Build history of the part. All positions in model axes, mm. Face numbers are marked on the shaded views. A direction names the side the tool comes from. Round coordinates to 2 decimals unless told otherwise and drop trailing zeros. Loops run counter-clockwise (first coordinate to the right, second up) from the corner with the lowest first, then second, coordinate; pieces in that order, holes last. Notation, with made-up numbers: (3.5, 85.25) - (44.5, 85.25) arc R32 cw to (44.5, 117.25) - close; hole circle Ø7 at (18, 64.25). An arc over 180 degrees is marked (long way). Put each result on its own line as item: value. Start each with the question number.
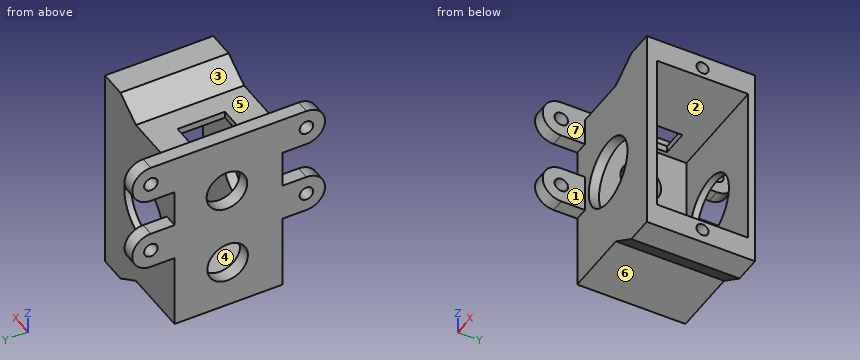
from build123d import *

# Parameters (mm, degrees)
P_IDAT_VYSUNUT_M1_DEPTH   = 15
P_IDAT_VYSUNUT_M2_DEPTH   = 15
SKICA10_W                 = 16
SKICA10_H                 = 24
ODEBRAT_VYSUNUT_M7_DEPTH  = 13.5
SKICA11_W                 = 2.5
SKICA11_H                 = 15
P_IDAT_VYSUNUT_M3_DEPTH   = 4
SKICA12_R                 = 0.9
ODEBRAT_VYSUNUT_M8_DEPTH  = 4
SKICA13_W                 = 4
SKICA13_H                 = 7
ODEBRAT_VYSUNUT_M9_DEPTH  = 4
SKICA17_W                 = 38.25
SKICA17_H                 = 32.5
ODEBRAT_VYSUNUT_M10_DEPTH = 16
P_IDAT_VYSUNUT_M4_DEPTH   = 1
SKICA20_R                 = 1
P_IDAT_VYSUNUT_M5_DEPTH   = 2
SKICA21_R                 = 5
ODEBRAT_VYSUNUT_M11_DEPTH = 22
LINPOLE1_COUNT            = 2
LINPOLE1_PITCH            = 11
SKICA22_R                 = 3
ODEBRAT_VYSUNUT_M12_DEPTH = 5
P_IDAT_VYSUNUT_M6_DEPTH   = 16
SKICA24_W                 = 2
SKICA24_H                 = 1.5
P_IDAT_VYSUNUT_M7_DEPTH   = 16


with BuildPart() as part:
    # Skica1 → Přidat vysunutím1 (new body)
    with BuildSketch(Plane(origin=(0, 0, 0), x_dir=(1, 0, 0), z_dir=(0, 1, 0))):
        Polygon((0, -11), (0, 11), (-3.25, 14.25), (-30.25, 14.25), (-30.25, 16.25), (-2.421572875, 16.25), (2, 11.828427125), (2, -11.828427125), (-2.421572875, -16.25), (-30.25, -16.25), (-30.25, -14.25), (-3.25, -14.25), align=None)
    extrude(amount=P_IDAT_VYSUNUT_M1_DEPTH)

    # Skica8 → Přidat vysunutím2 (add)
    with BuildSketch(Plane.XZ):
        Polygon((-0.343145751, 14.171572875), (26, 14.171572875), (26, -11.828427125), (2, -11.828427125), (2, 11.828427125), align=None)
    extrude(amount=-P_IDAT_VYSUNUT_M2_DEPTH)

    # Skica10 → Odebrat vysunutím7 (cut)
    with BuildSketch(Plane(origin=(0, 15, 0), x_dir=(1, 0, 0), z_dir=(0, 1, 0))):
        with Locations((18, -1.171572875)):
            Rectangle(SKICA10_W, SKICA10_H)
    extrude(amount=-ODEBRAT_VYSUNUT_M7_DEPTH, mode=Mode.SUBTRACT)

    # Skica11 → Přidat vysunutím3 (add)
    with BuildSketch(Plane(origin=(26, 0, 0), x_dir=(0, 0, -1), z_dir=(1, 0, 0))):
        with Locations((-15.421572875, 7.5)):
            Rectangle(SKICA11_W, SKICA11_H)
        with Locations((13.078427125, 7.5)):
            Rectangle(SKICA11_W, SKICA11_H)
    extrude(amount=-P_IDAT_VYSUNUT_M3_DEPTH)

    # Skica12 → Odebrat vysunutím8 (cut)
    with BuildSketch(Plane(origin=(26, 0, 0), x_dir=(0, 0, -1), z_dir=(1, 0, 0))):
        with Locations((-14.730217843, 8.25)):
            Circle(SKICA12_R)
        with Locations((12.269782157, 8.25)):
            Circle(SKICA12_R)
    extrude(amount=-ODEBRAT_VYSUNUT_M8_DEPTH, mode=Mode.SUBTRACT)

    # Skica13 → Odebrat vysunutím9 (cut)
    with BuildSketch(Plane.XY.offset(14.171572875)):
        with Locations((12.656854249, 8.25)):
            Rectangle(SKICA13_W, SKICA13_H)
    extrude(amount=-ODEBRAT_VYSUNUT_M9_DEPTH, mode=Mode.SUBTRACT)

    # Skica17 → Odebrat vysunutím10 (cut, through all)
    with BuildSketch(Plane(origin=(0, 15, 0), x_dir=(1, 0, 0), z_dir=(0, 1, 0))):
        with Locations((-11.125, 0)):
            Rectangle(SKICA17_W, SKICA17_H)
    extrude(amount=-ODEBRAT_VYSUNUT_M10_DEPTH, mode=Mode.SUBTRACT)

    # Skica19 → Přidat vysunutím4 (add)
    with BuildSketch(Plane(origin=(0, 15, 0), x_dir=(1, 0, 0), z_dir=(0, 1, 0))):
        Polygon((8, 11.828427125), (22, 11.828427125), (22, 14.328427125), (26, 14.328427125), (26, -16.671572875), (22, -16.671572875), (22, -14.171572875), (8, -14.171572875), align=None)
    extrude(amount=P_IDAT_VYSUNUT_M4_DEPTH)

    # Skica20 → Přidat vysunutím5 (add)
    with BuildSketch(Plane.ZY.offset(-8)):
        with BuildLine():
            Line((10.171572875, -3.5), (10.171572875, 0))
            Line((10.171572875, 0), (15.671572875, 0))
            Line((15.671572875, 0), (15.671572875, -3.5))
            ThreePointArc((15.671572875, -3.5), (12.921572875, -6.25), (10.171572875, -3.5))
        make_face()
        with Locations((12.921572875, -3.5)):
            Circle(SKICA20_R, mode=Mode.SUBTRACT)
        with BuildLine():
            Line((10.171572875, 16), (15.671572875, 16))
            Line((15.671572875, 16), (15.671572875, 19.5))
            ThreePointArc((15.671572875, 19.5), (12.921572875, 22.25), (10.171572875, 19.5))
            Line((10.171572875, 19.5), (10.171572875, 16))
        make_face()
        with Locations((12.921572875, 19.5)):
            Circle(SKICA20_R, mode=Mode.SUBTRACT)
    p_idat_vysunut_m5 = extrude(amount=-P_IDAT_VYSUNUT_M5_DEPTH)

    # Skica21 → Odebrat vysunutím11 (cut)
    with BuildSketch(Plane(origin=(0, 16, 0), x_dir=(1, 0, 0), z_dir=(0, 1, 0))):
        with Locations((16, -1.171572875)):
            Circle(SKICA21_R)
    extrude(amount=-ODEBRAT_VYSUNUT_M11_DEPTH, mode=Mode.SUBTRACT)

    # LinPole1: Přidat vysunutím5 ×2
    with Locations(*[(0, 0, -i * LINPOLE1_PITCH) for i in range(1, LINPOLE1_COUNT)]):
        add(p_idat_vysunut_m5)

    # Skica22 → Odebrat vysunutím12 (cut)
    with BuildSketch(Plane(origin=(10, 0, 0), x_dir=(0, 0, -1), z_dir=(1, 0, 0))):
        with Locations((-7.230444291, 8.25)):
            Circle(SKICA22_R)
        with Locations((4.769102832, 8.145746213)):
            Circle(SKICA22_R)
    extrude(amount=-ODEBRAT_VYSUNUT_M12_DEPTH, mode=Mode.SUBTRACT)

    # Skica23 → Přidat vysunutím6 (add)
    with BuildSketch(Plane(origin=(0, 16, 0), x_dir=(1, 0, 0), z_dir=(0, 1, 0))):
        Polygon((22, 14.328427125), (18, 11.828427125), (22, 11.828427125), align=None)
        Polygon((22, -14.171572875), (18, -14.171572875), (22, -16.671572875), align=None)
    extrude(amount=-P_IDAT_VYSUNUT_M6_DEPTH)

    # Skica24 → Přidat vysunutím7 (add)
    with BuildSketch(Plane.XZ.offset(-16)):
        with Locations((9, 14.921572875)):
            Rectangle(SKICA24_W, SKICA24_H)
    extrude(amount=P_IDAT_VYSUNUT_M7_DEPTH)


solid = part.part
Item 1: Which spindle directions (+Z, -Z, +X, -X, +Y, -Y) get a long thin tool onto all of the face, cutting with end or side? Do the marked faces 4, 5, 6 and 7. Say none if no direction does.
Item 2: Slice it at B-B (x = 16). Give the cut face in (y, z).
Item 3: Two-plate mould, pull along X, no slides. Class the marked faces 1, 2 and 3: pulls with the +X half, pulls with the -X half, needs draft (parallel to the pull), parting line crosses it, or undercut.
Item 4: Slice it at D-D (x = 13.5). Give the cut face in (y, z), plus the area to 3 significant figures.
Item 5: Slice it at A-A (x = 23). Give the cut face in (y, z).
Item 6: Drop flat-ended pins along their axis: pin 1 Ø2 at (x, y) = (9, -1.5) entering from +Z; pin 2 Ø10 at (x, z) = (20, 6.5) entering from +Y; pin 3 Ø2 at (y, z) = (8, -12.5) entering from +X; pin 4 Ø8 at (x, y) = (12, 8.5) entering from -Z. Give the stop position or say it passes through.
Item 7: Slice it at C-C (z = 11). Give the cut face in (x, y), plus the area to 3 significant figures.
Item 8: Drill centre lines: probe 1 along Z at (x, y) = (23.95, 8.25); probe 2 along Z at (x, y) = (25, 9.25); probe 3 along Z at (x, y) = (12.75, 13). Where is each one in solid material? Low to high. Write a range as [from, to].
Computed values:
1. face 4: +X
1. face 5: +Z, +Y, -Y
1. face 6: -Z, -X, +Y, -Y
1. face 7: +Z
2. outline: (0, -11.83) - (16, -11.83) - (16, -3.83) - (15, -3.83) - (15, -10.83) - (1.5, -10.83) - (1.5, -3.83) - (0, -3.83) - close; (0, 6.17) - (1.5, 6.17) - (1.5, 13.17) - (15, 13.17) - (15, 6.17) - (16, 6.17) - (16, 14.17) - (0, 14.17) - close
3. face 1: pulls with the +X half
3. face 2: needs draft
3. face 3: undercut
4. outline: (0, -11.83) - (16, -11.83) - (16, -3.16) - (15, -3.16) - (15, -10.83) - (1.5, -10.83) - (1.5, -3.16) - (0, -3.16) - close; (0, 5.5) - (1.5, 5.5) - (1.5, 13.17) - (4.75, 13.17) - (4.75, 14.17) - (0, 14.17) - close; (11.75, 13.17) - (15, 13.17) - (15, 5.5) - (16, 5.5) - (16, 14.17) - (11.75, 14.17) - close
4. area: 63.3 mm^2
5. outline: (0, -14.33) - (16, -14.33) - (16, 16.67) - (0, 16.67) - close; hole (1.5, -10.83) - (15, -10.83) - (15, 13.17) - (1.5, 13.17) - close; hole circle Ø1.8 at (8.25, -12.27); hole circle Ø1.8 at (8.25, 14.73)
6. pin 1: stops at z = 15.67
6. pin 2: stops at y = 16
6. pin 3: stops at x = 26
6. pin 4: stops at z = -11.83
7. outline: (8, -5.47) - (10, -5.47) - (10, 0) - (26, 0) - (26, 1.5) - (10, 1.5) - (10, 15) - (26, 15) - (26, 16) - (10, 16) - (10, 21.47) - (8, 21.47) - close
7. area: 93.9 mm^2
8. probe 1: z = [-14.33, -13.17], [-11.37, -10.83], [13.17, 13.83], [15.63, 16.67]
8. probe 2: z = [-14.33, -10.83], [13.17, 16.67]
8. probe 3: z = [-11.83, -10.83], [13.17, 14.17]
